Part model, mm, in its own coordinate system. Round coordinates to 2 decimals unless told otherwise and drop trailing zeros. Loops run counter-clockwise (first coordinate to the right, second up) from the corner with the lowest first, then second, coordinate; pieces in that order, holes last. Notation, with made-up numbers: (25.5, 8) -> (43.5, 8) arc R23 cw to (43.5, 36) -> close; hole circle Ø1 at (57, -34.75). An arc over 180 degrees is marked (long way). Answer as CSV lines item,"result".
Autodesk Inventor part; units mm, degrees
ref_plane "YZ Plane" through (0, 0, 0) normal (1, 0, 0) x (0, 1, 0)
ref_plane "XZ Plane" through (0, 0, 0) normal (0, 1, 0) x (-1, 0, 0)
ref_plane "XY Plane" through (0, 0, 0) normal (0, 0, 1) x (1, 0, 0)
sketch "Sketch1" plane through (0, 0, 0) normal (0, 0, 1) x (1, 0, 0)
  line L0 (23.8989, 56.2562) -> (111.3989, 56.2562)
  line L1 (111.3989, 56.2562) -> (111.3989, 26.2562)
  line L2 (111.3989, 26.2562) -> (23.8989, 26.2562)
  line L3 (21.3989, 28.7562) -> (21.3989, 53.7562)
  line L4 (21.3989, 53.7562) -> (23.8989, 56.2562)
  line L5 (21.3989, 28.7562) -> (23.8989, 26.2562)
  point P0 (0, 0)
  point P1 (21.3989, 56.2562)
  point P2 (21.3989, 26.2562)
  dimension "d0" = 30
  dimension "d1" = 90
  dimension "d2" = 2.5
  dimension "d3" = 2.5
  dimension "d4" = 2.5
  dimension "d5" = 2.5
extrude "Extrusion1" add sketch "Sketch1" along normal blind 7
sketch "Sketch2" plane through (0, 0, 7) normal (0, 0, 1) x (1, 0, 0)
  line L0 (111.3989, 26.2562) -> (111.3989, 56.2562) construction
  line L1 (111.3989, 41.2562) -> (21.3989, 41.2562) construction
  line L2 (21.3989, 53.7562) -> (21.3989, 28.7562) construction
  line L3 (23.8989, 26.2562) -> (111.3989, 26.2562)
  point P0 (0, 0)
  point P1 (26.3989, 31.2562)
  point P2 (26.3989, 51.2562)
  dimension "d8" = 5
  dimension "d9" = 5
hole "Hole1" at (26.3989, 31.2562, 7) at (26.3989, 51.2562, 7) direction (0, 0, -1) diameter 4 end through all
sketch "Sketch3" plane through (0, 0, 7) normal (0, 0, 1) x (1, 0, 0)
  circle A0 centre (67.6489, 41.2562) radius 12.5 construction
  line L0 (21.3989, 53.7562) -> (21.3989, 28.7562)
  line L1 (21.3989, 41.2562) -> (111.3989, 41.2562) construction
  line L2 (111.3989, 26.2562) -> (111.3989, 56.2562)
  line L3 (23.8989, 26.2562) -> (111.3989, 26.2562) construction
  line L4 (67.6489, 26.2562) -> (67.6489, 56.2562) construction
  point P0 (0, 0)
  dimension "d17" = 25
properties part number "Dedo" material "MDF Medium Density Fiberboard"
Q1. Saw through at A-A, the plane y = 50.75. Write the cut outline in (x, z), then the cut area to 3 significant figures.
Geometry results:
outline,"(21.4, 0) -> (24.46, 0) -> (24.46, 7) -> (21.4, 7) -> close; (28.33, 0) -> (111.4, 0) -> (111.4, 7) -> (28.33, 7) -> close"
area,"603 mm2"
Q2. Two-plate mould, pull along X, no slides. Class faces 1 (the face through (22.631, 27.524, 3.451)), 2 (the face through (111.399, 41, 3)), 3 (the face through (25.8, 49.35, 3.45)), 4 (the face through (66, 41, 0)): pulls with the +X half, pulls with the -X half, needs draft (parallel to the pull), parting line crosses it, or undercut.
Geometry results:
face 1,"pulls with the -X half"
face 2,"pulls with the +X half"
face 3,"undercut"
face 4,"needs draft"
Q3. Drill centre lines: line 1 along X through (y, z) = (31.5, 1); line 2 along X through (y, z) = (33, 1); line 3 along X through (y, z) = (54.75, 2.5). Where is each one in solid material? Low to high.
Geometry results:
line 1,"21.4 to 24.41, 28.38 to 111.4"
line 2,"21.4 to 25.42, 27.38 to 111.4"
line 3,"22.39 to 111.4"
Q4. Drop a flat-ended pin along its axis: P1, Ø12, axis at x = 91, y = 38, coming from the -Z side. Give the stop position or say it passes through.
Geometry results:
P1,"z = 0"
